Can you work these out from the model? Positions are in its coordinate system, mm. A direction names the side the tool comes from. Coordinates: 2 decimals unless noted, no trailing zeros. Order: outer loops, then holes, each group sorted by start corner. A loop starts at its lowest first (then second) coordinate and runs counter-clockwise, first axis right, second up. Notation, with made-up numbers: (86, 36.5) - (141, 36.5) arc R25 cw to (141, 70.5) - close; hole circle Ø3 at (38.5, -32). An arc over 180 degrees is marked (long way). Return JSON: item names as keys, results as strings. Group by question number.
1) If I drill on line 1 along Z through (x, y) = (-2.25, -8); line 2 along Z through (x, y) = (9.75, 6); line 3 along X through (y, z) = (-1, 5), over which ranges is the centre line in solid material (lowest first)?
2) Imagine slicing it at A-A (y = -8). Write out the boundary of the cut face in (x, z).
3) Imagine slicing it at D-D (z = 5). Write out the boundary of the cut face in (x, y), and give its area (3 significant figures).
4) Imagine slicing it at C-C (x = 2.75). Write out the boundary of the cut face in (y, z).
5) Which directions (+Z, -Z, +X, -X, +Y, -Y) give clear straight access to the entire face, cutting with the end or side of a thin tool? Please do faces 1 (the face through (-8, 0, 7)), 2 (the face through (7.07, 5.263, 5.676)), 3 (the face through (1.43, -12.35, 5.45)), 4 (the face through (-12, -2, 5)).
6) Imagine slicing it at B-B (x = 0). Write out the boundary of the cut face in (y, z).
7) If we mould it in two halves opening along Y, with no side actions, what happens to faces 5 (the face through (12, -2, 5)), 6 (the face through (2, 6, 5)), 7 (the face through (0, 10, 5)), 8 (the face through (0, -14, 3))? For each: pulls with the +Y half, pulls with the -Y half, needs draft (parallel to the pull), parting line crosses it, or undercut.
8) For pin 1 Ø0.9 at (x, y) = (-8.5, 0.5) entering from -Z; pin 2 Ø2.5 at (x, z) = (0, 5) entering from -Y, each with a flat end and sliding along its axis, tell me the tip position at first contact or that it passes through.
```python
from build123d import *

# Parameters (mm, degrees)
SKETCH_W        = 24
SKETCH_H        = 24
SKETCH_R        = 4
PAD_DEPTH       = 10
SKETCH002_R     = 3.05
POCKET_DEPTH    = 24.001
SKETCH003_R     = 1
POCKET001_DEPTH = 10
SKETCH004_R     = 1.5
POCKET002_DEPTH = 7
SKETCH005_R     = 1.5
POCKET003_DEPTH = 5


with BuildPart() as part:
    # Sketch → Pad (new body)
    with BuildSketch(Plane.XY):
        with Locations((0, -2)):
            Rectangle(SKETCH_W, SKETCH_H)
        Circle(SKETCH_R, mode=Mode.SUBTRACT)
    extrude(amount=PAD_DEPTH)

    # Sketch002 → Pocket (cut, through all)
    with BuildSketch(Plane.YZ.offset(12)):
        with Locations((-8, 5)):
            Circle(SKETCH002_R)
    extrude(amount=-POCKET_DEPTH, mode=Mode.SUBTRACT)

    # Sketch003 (on Face3 of Pocket) → Pocket001 (cut)
    with BuildSketch(Plane.YZ.offset(12)):
        with Locations((6, 5)):
            Circle(SKETCH003_R)
    extrude(amount=-POCKET001_DEPTH, mode=Mode.SUBTRACT)

    # Sketch004 (on Face4 of Pocket001) → Pocket002 (cut)
    with BuildSketch(Plane(origin=(0, 0, 0), x_dir=(1, 0, 0), z_dir=(0, 0, -1))):
        with Locations((8, -0.003153)):
            Circle(SKETCH004_R)
        with Locations((-8, -0.04227)):
            Circle(SKETCH004_R)
    extrude(amount=-POCKET002_DEPTH, mode=Mode.SUBTRACT)

    # Sketch005 (on Face6 of Pocket002) → Pocket003 (cut)
    with BuildSketch(Plane.XZ.offset(14)):
        with Locations((0, 5)):
            Circle(SKETCH005_R)
    extrude(amount=-POCKET003_DEPTH, mode=Mode.SUBTRACT)


solid = part.part
```
Calculated:
{
 "1": {"line 1": "0 to 1.95, 8.05 to 10", "line 2": "0 to 4, 6 to 10", "line 3": "-12 to -9.08, -6.92 to -3.87, 3.87 to 6.88, 9.12 to 12"},
 "2": {"outline": "(-12, 0) - (12, 0) - (12, 1.95) - (-12, 1.95) - close; (-12, 8.05) - (12, 8.05) - (12, 10) - (-12, 10) - close"},
 "3": {"outline": "(-12, -14) - (-1.5, -14) - (-1.5, -11.05) - (-12, -11.05) - close; (-12, -4.95) - (12, -4.95) - (12, 5) - (2, 5) - (2, 7) - (12, 7) - (12, 10) - (-12, 10) - close; (1.5, -14) - (12, -14) - (12, -11.05) - (1.5, -11.05) - close; hole circle Ø3 at (-8, 0.04); hole circle Ø8 at (0, 0); hole circle Ø3 at (8, 0)", "area": "336 mm2"},
 "4": {"outline": "(-14, 0) - (-2.9, 0) - (-2.9, 10) - (-14, 10) - close; (2.9, 0) - (10, 0) - (10, 10) - (2.9, 10) - close; hole circle Ø6.1 at (-8, 5); hole circle Ø2 at (6, 5)"},
 "5": {"face 1": "-Z", "face 2": "+X", "face 3": "-Y", "face 4": "+Z, -Z, -X, +Y, -Y"},
 "6": {"outline": "(-14, 0) - (-4, 0) - (-4, 10) - (-14, 10) - (-14, 6.5) - (-10.66, 6.5) arc R3.05 cw (long way) to (-10.66, 3.5) - (-14, 3.5) - close; (4, 0) - (10, 0) - (10, 10) - (4, 10) - close"},
 "7": {"face 5": "needs draft", "face 6": "undercut", "face 7": "pulls with the +Y half", "face 8": "pulls with the -Y half"},
 "8": {"pin 1": "z = 7", "pin 2": "y = -5.22"}
}
